Autodesk Inventor part; units mm, degrees
ref_plane "YZ Plane" through (0, 0, 0) normal (1, 0, 0) x (0, 1, 0)
ref_plane "XZ Plane" through (0, 0, 0) normal (0, 1, 0) x (-1, 0, 0)
ref_plane "XY Plane" through (0, 0, 0) normal (0, 0, 1) x (1, 0, 0)
sketch "Sketch1" plane through (0, 0, 0) normal (0, 1, 0) x (-1, 0, 0)
  line L0 (127.8939, 73.8396) -> (127.8939, -73.8396)
  line L1 (127.8939, -73.8396) -> (0, -147.6791)
  line L2 (0, -147.6791) -> (-127.8939, -73.8396)
  line L3 (-127.8939, -73.8396) -> (-127.8939, 73.8396)
  line L4 (-127.8939, 73.8396) -> (0, 147.6791)
  line L5 (0, 147.6791) -> (127.8939, 73.8396)
  line L6 (-18, 10.3923) -> (0, 20.7846)
  line L7 (0, 20.7846) -> (18, 10.3923)
  line L8 (18, 10.3923) -> (18, -10.3923)
  line L9 (18, -10.3923) -> (0, -20.7846)
  line L10 (0, -20.7846) -> (-18, -10.3923)
  line L11 (-18, -10.3923) -> (-18, 10.3923)
  point P0 (0, 0)
  point P1 (0, 0)
  point P2 (0, 0)
  dimension "Shex" = 36
extrude "Extrusion1" add sketch "Sketch1" along normal blind 15 contours L6 L7 L8 L9 L10 L11
sketch "Sketch2" plane through (0, 0, 0) normal (1, 0, 0) x (0, 1, 0)
  line L0 (0, -20.7846) -> (15, -20.7846) construction
  line L1 (15, -20.7846) -> (13.3923, -20.7846)
  line L2 (13.3923, -20.7846) -> (15, -18)
  line L3 (15, -18) -> (15, -20.7846)
  line L4 (-3, 0) -> (18, 0)
  point P0 (0, 0)
  dimension "d4" = 60
  dimension "d5" = 36
revolve "Revolution1" cut sketch "Sketch2" angle 360 about axis through (0, -10, 0) along (0, 1, 0)
sketch "Sketch3" plane through (0, 0, 0) normal (0, 0, 1) x (1, 0, 0)
  line L0 (0, 0) -> (12, 0)
  line L1 (12, 0) -> (12, -120)
  line L2 (12, -120) -> (0, -120)
  line L3 (0, -120) -> (0, 0)
  dimension "L" = 120
  dimension "Dia" = 24
revolve "Revolution2" add sketch "Sketch3" angle 360 about axis through (0, -120, 0) along (0, 1, 0)
fillet "Fillet1" radius 0.8 1 edges at (-12, 0, 0)
chamfer "Chamfer1" distance 2 angle 45 1 edges at (-12, -120, 0)
thread "Thread2"
sketch "Sketch6" plane through (0, 0, 0) normal (1, 0, 0) x (0, 1, 0)
  line L0 (-147, 0) -> (42, 0)
  line L1 (0, -20.7846) -> (13.3923, -20.7846)
  line L2 (0, -20.7846) -> (0, -10.3923)
  line L3 (0, -10.3923) -> (13.3923, -10.3923)
  line L4 (0, -20.7846) -> (0.5, -20.7846)
  line L5 (0.5, -20.7846) -> (0.5, -18)
  line L6 (0.5, -18) -> (0, -18)
  line L7 (0, -18) -> (0, -20.7846)
  point P0 (0, 0)
  point P1 (15, -15.5885)
  point P2 (0, -18)
  dimension "a" = 0.5
  dimension "d34" = 36
revolve "Revolution3" cut sketch "Sketch6" angle 360 about axis through (0, -10, 0) along (0, 1, 0)
equation "\"d5\" = Shex"
equation "\"d31\" = b - cham"
equation "\"d34\" = Shex"
equation "\"b\" = 56"
properties part number "Part16 Real Bolt Thread" material "Steel"
The listing builds one solid part. Answer for the finished solid, in the listing's coordinates (mm). A direction names the side the tool comes from. Give positions to 0.01 mm unless a question says otherwise; leave off trailing zeros. Loops run counter-clockwise (first coordinate to the right, second up) from the corner with the lowest first, then second, coordinate; pieces in that order, holes last. Notation, with made-up numbers: M 27,-1 L 46,-1 A4 cw 46,3 Z; hole C -33,78 d4. An arc over 180 degrees is marked long. One line per item, written item: value.
Q1. A cutting plane is placed at A-A on y = -88. Determine the outline of the cut face in (x, z).
Working result:
outline: C 0,0 d24
Q2. For faces 1 (the face through (0, 0.5, -19)), 2 (the face through (12.3, 0, 4.3)), 3 (the face through (16, 0.5, -9)), 4 (the face through (16, 0.5, 9)), determine the directions among +Z, -Z, +X, -X, +Y, -Y from which every point of the face is accessible in a straight line to the end or side of a thin tool.
Working result:
face 1: -Z, -Y
face 2: -Y
face 3: -Z, +X, -Y
face 4: +Z, +X, -Y
Q3. Find the intervals of material crossed by line 1 (Y direction, x = 3.5, z = -15); line 2 (Z direction, x = 1.5, y = -53); line 3 (Z direction, x = 1.5, y = 2), in increasing order. Write a range as from..to.
Working result:
line 1: y = 0..15
line 2: z = -11.91..11.91
line 3: z = -19.92..19.92
Q4. Flat-ended cylindrical pins translate along their axes: P1, Ø4, axis at y = -72.5, z = 4, coming from the -X side; P2, Ø10, axis at x = 12.5, z = -10, coming from the -Y side; P3, Ø2, axis at y = -23, z = -6, coming from the +X side. Find the tip coordinate at first contact, or state that the pin passes through.
Working result:
P1: stops at x = -11.83
P2: stops at y = -118.99
P3: stops at x = 10.91
